```python
from build123d import *

# Parameters (mm, degrees)
SKETCH_W        = 150
SKETCH_H        = 100
PAD_DEPTH       = 5
SKETCH001_W     = 23
SKETCH001_H     = 12
POCKET_DEPTH    = 16
SKETCH002_R     = 0.85
SKETCH002_R_2   = 3.5
SKETCH002_W     = 120
SKETCH002_H     = 50
POCKET001_DEPTH = 10
SKETCH003_R     = 3.5
POCKET002_DEPTH = 10
FILLET_R        = 9
FILLET001_R     = 9
FILLET002_R     = 9
FILLET003_R     = 9


with BuildPart() as part:
    # Sketch → Pad (new body)
    with BuildSketch(Plane.XY):
        Rectangle(SKETCH_W, SKETCH_H)
    extrude(amount=PAD_DEPTH)

    # Sketch001 (on Face6 of Pad) → Pocket (cut)
    with BuildSketch(Plane.XY.offset(5)):
        with Locations((-53.5, 44)):
            Rectangle(SKETCH001_W, SKETCH001_H)
        with Locations((-53.5, -44)):
            Rectangle(SKETCH001_W, SKETCH001_H)
        with Locations((0, 44)):
            Rectangle(SKETCH001_W, SKETCH001_H)
        with Locations((0, -44)):
            Rectangle(SKETCH001_W, SKETCH001_H)
        with Locations((53.5, 44)):
            Rectangle(SKETCH001_W, SKETCH001_H)
        with Locations((53.5, -44)):
            Rectangle(SKETCH001_W, SKETCH001_H)
    extrude(amount=-POCKET_DEPTH, mode=Mode.SUBTRACT)

    # Sketch002 (on Face4 of Pocket) → Pocket001 (cut)
    with BuildSketch(Plane.XY.offset(5)):
        with Locations((-39.85, -44.1)):
            Circle(SKETCH002_R)
        with Locations((-67.15, 44.1)):
            Circle(SKETCH002_R)
        with Locations((-39.85, 44.1)):
            Circle(SKETCH002_R)
        with Locations((-13.65, 44.1)):
            Circle(SKETCH002_R)
        with Locations((13.65, 44.1)):
            Circle(SKETCH002_R)
        with Locations((39.85, 44.1)):
            Circle(SKETCH002_R)
        with Locations((67.15, 44.1)):
            Circle(SKETCH002_R)
        with Locations((39.85, -44.1)):
            Circle(SKETCH002_R)
        with Locations((67.15, -44.1)):
            Circle(SKETCH002_R)
        with Locations((13.65, -44.1)):
            Circle(SKETCH002_R)
        with Locations((-13.65, -44.1)):
            Circle(SKETCH002_R)
        with Locations((-67.15, -44.1)):
            Circle(SKETCH002_R)
        with Locations((67.5, 30)):
            Circle(SKETCH002_R_2)
        with Locations((67.5, -30)):
            Circle(SKETCH002_R_2)
        with Locations((-67.5, 30)):
            Circle(SKETCH002_R_2)
        with Locations((-67.5, -30)):
            Circle(SKETCH002_R_2)
        Rectangle(SKETCH002_W, SKETCH002_H)
    extrude(amount=-POCKET001_DEPTH, mode=Mode.SUBTRACT)

    # Sketch003 → Pocket002 (cut)
    with BuildSketch(Plane.XY.offset(7)):
        with Locations((-26, -42.5)):
            Circle(SKETCH003_R)
        with Locations((27.5, -42.5)):
            Circle(SKETCH003_R)
        with Locations((-26, 42.5)):
            Circle(SKETCH003_R)
        with Locations((27.5, 42.5)):
            Circle(SKETCH003_R)
    extrude(amount=-POCKET002_DEPTH, mode=Mode.SUBTRACT)

    # Fillet
    fillet_edges = [part.edges().sort_by_distance(p)[0] for p in [
        (75, -50, 2.5),
    ]]
    fillet(fillet_edges, radius=FILLET_R)

    # Fillet001
    fillet001_edges = [part.edges().sort_by_distance(p)[0] for p in [
        (75, 50, 2.5),
    ]]
    fillet(fillet001_edges, radius=FILLET001_R)

    # Fillet002
    fillet002_edges = [part.edges().sort_by_distance(p)[0] for p in [
        (-75, 50, 2.5),
    ]]
    fillet(fillet002_edges, radius=FILLET002_R)

    # Fillet003
    fillet003_edges = [part.edges().sort_by_distance(p)[0] for p in [
        (-75, -50, 2.5),
    ]]
    fillet(fillet003_edges, radius=FILLET003_R)


solid = part.part
```
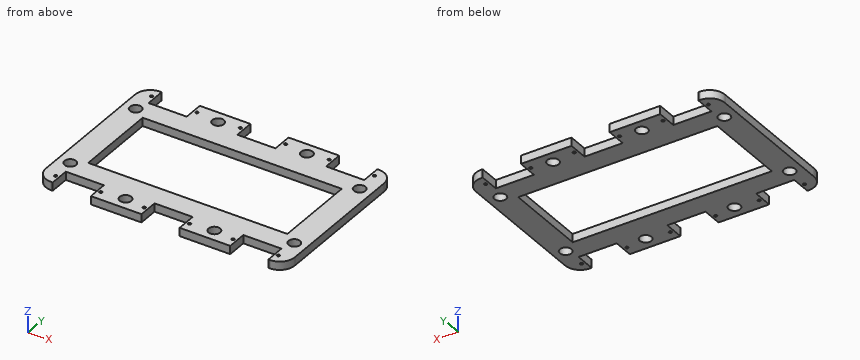
Model file for the job. Use its own axes, mm. Round coordinates to 2 decimals unless told otherwise and drop trailing zeros. Write each loop counter-clockwise with the first axis right and the second up, starting at its lowest first coordinate (ties: lowest second). Pieces come first, ordered by that corner, then holes. Notation, with made-up numbers: (32.25, 16) - (82.25, 16) arc R20 cw to (82.25, 48) - close; hole circle Ø4 at (87, -27.75). An arc over 180 degrees is marked (long way). One line per item, written item: value.
(1) Cut at A-A, the plane y = 10. Give the cut face in (x, z).
Values follow:
outline: (-75, 0) - (-60, 0) - (-60, 5) - (-75, 5) - close; (60, 0) - (75, 0) - (75, 5) - (60, 5) - close
(2) Wall check: probe 1 along Y at (x, z) = (39.85, 3.15); probe 2 along Y at (x, z) = (27.5, 3.1); probe 3 along Y at (x, z) = (7, 3.4). Give the ranges that are in metal, low to high.
Values follow:
probe 1: y = -50 to -44.95, -43.25 to -25, 25 to 43.25, 44.95 to 50
probe 2: y = -50 to -46, -39 to -25, 25 to 39, 46 to 50
probe 3: y = -38 to -25, 25 to 38
(3) Cut at B-B, the plane x = -7. Give the cut face in (y, z), plus the area to 3 significant figures.
Values follow:
outline: (-38, 0) - (-25, 0) - (-25, 5) - (-38, 5) - close; (25, 0) - (38, 0) - (38, 5) - (25, 5) - close
area: 130 mm²
(4) Cut at D-D, the plane y = 30. Give the cut face in (x, z).
Values follow:
outline: (-75, 0) - (-71, 0) - (-71, 5) - (-75, 5) - close; (-64, 0) - (64, 0) - (64, 5) - (-64, 5) - close; (71, 0) - (75, 0) - (75, 5) - (71, 5) - close
(5) Drop flat-ended pins along their axis: P1, Ø5.5, axis at x = 27.5, y = -42.5, coming from the +Z side; P2, Ø2.5, axis at y = -44, z = 1.5, coming from the +X side; P3, Ø1.5, axis at y = -46, z = 3.5, coming from the -X side; P4, Ø2.5, axis at x = 54.5, z = 2.5, coming from the +Y side. Give the stop position or say it passes through.
Values follow:
P1: passes through
P2: stops at x = 74.83
P3: stops at x = -73.93
P4: stops at y = 38
(6) Cut at C-C, the plane x = 27.5. Give the cut face in (y, z).
Values follow:
outline: (-50, 0) - (-46, 0) - (-46, 5) - (-50, 5) - close; (-39, 0) - (-25, 0) - (-25, 5) - (-39, 5) - close; (25, 0) - (39, 0) - (39, 5) - (25, 5) - close; (46, 0) - (50, 0) - (50, 5) - (46, 5) - close
